Autodesk Inventor part; units mm, degrees
ref_plane "YZ Plane" through (0, 0, 0) normal (1, 0, 0) x (0, 1, 0)
ref_plane "XZ Plane" through (0, 0, 0) normal (0, 1, 0) x (-1, 0, 0)
ref_plane "XY Plane" through (0, 0, 0) normal (0, 0, 1) x (1, 0, 0)
sketch "Sketch1" plane through (0, 0, 0) normal (0, 1, 0) x (-1, 0, 0)
  line L0 (-5, 25) -> (5, 25)
  line L1 (5, 25) -> (5, -25)
  line L2 (5, -25) -> (-5, -25)
  line L3 (-5, -25) -> (-5, 25)
  line L4 (-5, 25) -> (5, -25) construction
  line L5 (5, 25) -> (-5, -25) construction
  circle A0 centre (0, 10) radius 2.5
  line L6 (0, 0) -> (5, 0) construction
  circle A1 centre (0, -10) radius 2.5
  dimension "d0" = 10
  dimension "d1" = 5
  dimension "d2" = 10
  dimension "d3" = 50
extrude "Extrusion1" add sketch "Sketch1" along normal blind 5
fillet "Fillet1" radius 2 4 edges at (5, 2.5, 25) (5, 2.5, -25) (-5, 2.5, 25) (-5, 2.5, -25)
chamfer "Chamfer1" distance 2 angle 45 2 edges at (2.5, 5, -10) (2.5, 5, 10)
properties part number "Stop"
Part model, mm, in its own coordinate system. Coordinates: 2 decimals unless noted, no trailing zeros. Order: outer loops, then holes, each group sorted by start corner. A loop starts at its lowest first (then second) coordinate and runs counter-clockwise, first axis right, second up. Notation, with made-up numbers: (-18, 47) - (11, 47) arc R18 ccw to (11, 57) - close; hole circle Ø3 at (13, 8.25). An arc over 180 degrees is marked (long way). Return JSON: item names as keys, results as strings. Group by question number.
Item 1: Drill centre lines: probe 1 along Z at (x, y) = (0, 0.7); probe 2 along X at (y, z) = (4.4, -12.5); probe 3 along Z at (x, y) = (-0.5, 3.8). Where is each one in solid material? Low to high. Write a range as from..to.
Item 2: Cut at B-B (x = 0). List the corners of the cut face in (y, z), plus the area to 3 significant figures.
Item 3: Pull direction X, two halves, no side cores. Call faces 1 (the face through (4.4, 2.54, 24.43)), 2 (the face through (0, 5, 0)), 3 (the face through (-1.411, 3.125, 12.214)), 4 (the face through (0.54, 1.48, -7.56)): pulls with the +X half, pulls with the -X half, needs draft (parallel to the pull), parting line crosses it, or undercut.
Item 4: Cut at D-D (y = 1.45). List the corners of the cut face in (x, z), plus the area to 3 significant figures.
Item 5: Cut at A-A (y = 4.1). List the corners of the cut face in (x, z), plus the area to 3 significant figures.
Item 6: Cut at C-C (z = -10). List the corners of the cut face in (x, y).
Item 7: Pin check, flat tip, straight feed: pin 1 (2 mm diameter, centred on x = 0, z = -12.5, fed in from +Y). Stop position of the tip, or through.
Check values:
{
 "1": {"probe 1": "z = -25..-12.5, -7.5..7.5, 12.5..25", "probe 2": "x = -5..-2.99, 2.99..5", "probe 3": "z = -25..-13.26, -6.74..6.74, 13.26..25"},
 "2": {"outline": "(0, -25) - (5, -25) - (5, -14.5) - (3, -12.5) - (0, -12.5) - close; (0, -7.5) - (3, -7.5) - (5, -5.5) - (5, 5.5) - (3, 7.5) - (0, 7.5) - close; (0, 12.5) - (3, 12.5) - (5, 14.5) - (5, 25) - (0, 25) - close", "area": "192 mm2"},
 "3": {"face 1": "pulls with the +X half", "face 2": "needs draft", "face 3": "undercut", "face 4": "undercut"},
 "4": {"outline": "(-5, -23) arc R2 ccw to (-3, -25) - (3, -25) arc R2 ccw to (5, -23) - (5, 23) arc R2 ccw to (3, 25) - (-3, 25) arc R2 ccw to (-5, 23) - close; hole circle Ø5 at (0, -10); hole circle Ø5 at (0, 10)", "area": "457 mm2"},
 "5": {"outline": "(-5, -23) arc R2 ccw to (-3, -25) - (3, -25) arc R2 ccw to (5, -23) - (5, 23) arc R2 ccw to (3, 25) - (-3, 25) arc R2 ccw to (-5, 23) - close; hole circle Ø7.2 at (0, -10); hole circle Ø7.2 at (0, 10)", "area": "415 mm2"},
 "6": {"outline": "(-5, 0) - (-2.5, 0) - (-2.5, 3) - (-4.5, 5) - (-5, 5) - close; (2.5, 0) - (5, 0) - (5, 5) - (4.5, 5) - (2.5, 3) - close"},
 "7": {"pin 1": "stops at y = 4"}
}
